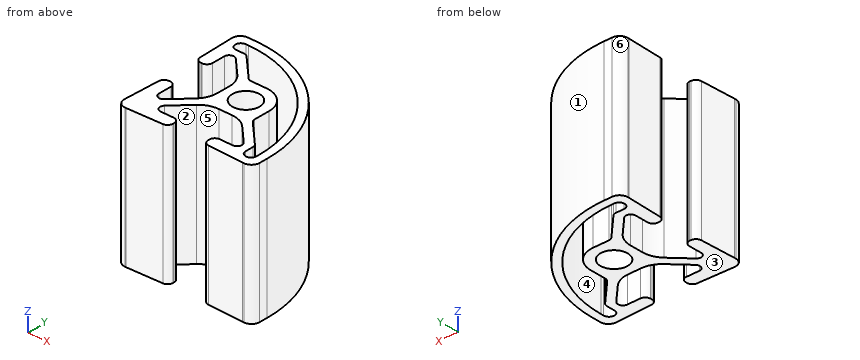
from build123d import *

# Parameters (mm, degrees)
SKETCH1_R      = 2.5
EXTRUDE1_DEPTH = 25.4


with BuildPart() as part:
    # Sketch1 → Extrude1 (new body)
    with BuildSketch(Plane.XY):
        with BuildLine():
            Line((1.22051236, -4.17896), (-1.22051236, -4.17896))
            ThreePointArc((-1.22051236, -4.17896), (-2.846916947, -4.502471987), (-4.22571618, -5.42375618))
            Line((-4.22571618, -5.42375618), (-7.286523897, -8.484563897))
            ThreePointArc((-7.286523897, -8.484563897), (-7.481619373, -9.465375089), (-6.650127794, -10.02096))
            Line((-6.650127794, -10.02096), (-4.24, -10.02096))
            ThreePointArc((-4.24, -10.02096), (-3.532893219, -10.313853219), (-3.24, -11.02096))
            Line((-3.24, -11.02096), (-3.24, -11.272405454))
            ThreePointArc((-3.24, -11.272405454), (-3.5206602, -11.967063824), (-4.205100503, -12.271796281))
            Line((-4.205100503, -12.271796281), (-10.74, -12.5))
            Line((-10.74, -12.5), (-11, -12.5))
            ThreePointArc((-11, -12.5), (-12.060660172, -12.060660172), (-12.5, -11))
            Line((-12.5, -11), (-12.5, -10.74))
            Line((-12.5, -10.74), (-12.271796281, -4.205100503))
            ThreePointArc((-12.271796281, -4.205100503), (-11.967063824, -3.5206602), (-11.272405454, -3.24))
            Line((-11.272405454, -3.24), (-11.02096, -3.24))
            ThreePointArc((-11.02096, -3.24), (-10.313853219, -3.532893219), (-10.02096, -4.24))
            Line((-10.02096, -4.24), (-10.02096, -6.650127794))
            ThreePointArc((-10.02096, -6.650127794), (-9.465375089, -7.481619373), (-8.484563897, -7.286523897))
            Line((-8.484563897, -7.286523897), (-5.42375618, -4.22571618))
            ThreePointArc((-5.42375618, -4.22571618), (-4.502471987, -2.846916947), (-4.17896, -1.22051236))
            Line((-4.17896, -1.22051236), (-4.17896, 1.22051236))
            ThreePointArc((-4.17896, 1.22051236), (-4.502471987, 2.846916947), (-5.42375618, 4.22571618))
            Line((-5.42375618, 4.22571618), (-8.484563897, 7.286523897))
            ThreePointArc((-8.484563897, 7.286523897), (-9.465375089, 7.481619373), (-10.02096, 6.650127794))
            Line((-10.02096, 6.650127794), (-10.02096, 4.24))
            ThreePointArc((-10.02096, 4.24), (-10.313853219, 3.532893219), (-11.02096, 3.24))
            Line((-11.02096, 3.24), (-11.272405454, 3.24))
            ThreePointArc((-11.272405454, 3.24), (-11.967063824, 3.5206602), (-12.271796281, 4.205100503))
            Line((-12.271796281, 4.205100503), (-12.5, 10.74))
            Line((-12.5, 10.74), (-12.5, 11))
            ThreePointArc((-12.5, 11), (-12.060660172, 12.060660172), (-11, 12.5))
            Line((-11, 12.5), (-9.5, 12.5))
            ThreePointArc((-9.5, 12.5), (6.056349186, 6.056349186), (12.5, -9.5))
            Line((12.5, -9.5), (12.5, -11))
            ThreePointArc((12.5, -11), (12.060660172, -12.060660172), (11, -12.5))
            Line((11, -12.5), (10.74, -12.5))
            Line((10.74, -12.5), (4.205100503, -12.271796281))
            ThreePointArc((4.205100503, -12.271796281), (3.5206602, -11.967063824), (3.24, -11.272405454))
            Line((3.24, -11.272405454), (3.24, -11.02096))
            ThreePointArc((3.24, -11.02096), (3.532893219, -10.313853219), (4.24, -10.02096))
            Line((4.24, -10.02096), (6.650127794, -10.02096))
            ThreePointArc((6.650127794, -10.02096), (7.481619373, -9.465375089), (7.286523897, -8.484563897))
            Line((7.286523897, -8.484563897), (4.22571618, -5.42375618))
            ThreePointArc((4.22571618, -5.42375618), (2.846916947, -4.502471987), (1.22051236, -4.17896))
        make_face()
        Circle(SKETCH1_R, mode=Mode.SUBTRACT)
        with BuildLine():
            Line((4.25, 0), (4.25, -2.912506094))
            ThreePointArc((4.25, -2.912506094), (4.326120467, -3.295189526), (4.542893219, -3.619612875))
            Line((4.542893219, -3.619612875), (8.707106781, -7.783826438))
            ThreePointArc((8.707106781, -7.783826438), (8.923879533, -8.108249786), (9, -8.490933219))
            Line((9, -8.490933219), (9, -10))
            ThreePointArc((9, -10), (10, -11), (11, -10))
            Line((11, -10), (11, -9.5))
            ThreePointArc((11, -9.5), (4.995689014, 4.995689014), (-9.5, 11))
            Line((-9.5, 11), (-10, 11))
            ThreePointArc((-10, 11), (-11, 10), (-10, 9))
            Line((-10, 9), (-8.490933219, 9))
            ThreePointArc((-8.490933219, 9), (-8.108249786, 8.923879533), (-7.783826438, 8.707106781))
            Line((-7.783826438, 8.707106781), (-3.619612875, 4.542893219))
            ThreePointArc((-3.619612875, 4.542893219), (-3.295189526, 4.326120467), (-2.912506094, 4.25))
            Line((-2.912506094, 4.25), (0, 4.25))
            ThreePointArc((0, 4.25), (3.00520382, 3.00520382), (4.25, 0))
        make_face(mode=Mode.SUBTRACT)
    extrude(amount=EXTRUDE1_DEPTH)


solid = part.part
The model under review builds one solid part; all positions refer to its coordinate system, in mm. Face numbers are marked on the shaded views. A direction names the side the tool comes from. Coordinates: 2 decimals unless noted, no trailing zeros. Write each loop counter-clockwise with the first axis right and the second up, starting at its lowest first coordinate (ties: lowest second). Pieces come first, ordered by that corner, then holes. Notation, with made-up numbers: (-4.75, 58.5) - (45.25, 58.5) arc R19 cw to (45.25, 69.5) - close; hole circle Ø1 at (-13, -13.75). An arc over 180 degrees is marked (long way). Answer as CSV lines item,"result".
(1) Clearance check with flat-ended pins moving along their axes: pin 1 Ø1.9 at (y, z) = (-6, 13.5) entering from +X; pin 2 Ø0.7 at (y, z) = (5, 11) entering from +X; pin 3 Ø1.9 at (x, z) = (-5, 13) entering from +Y; pin 4 Ø6 at (x, y) = (0, 0) entering from +Z. State where each tip first meets the part, or that it passes through.
Data:
pin 1,"stops at x = 12.35"
pin 2,"stops at x = 7.35"
pin 3,"stops at y = 12.21"
pin 4,"stops at z = 25.4"
(2) We need section B-B (x = -6.25). Give the boundary of the cut face in (y, z).
Data:
outline,"(-12.34, 0) - (-10.02, 0) - (-10.02, 25.4) - (-12.34, 25.4) - close; (-7.45, 0) - (-5.05, 0) - (-5.05, 25.4) - (-7.45, 25.4) - close; (5.05, 0) - (7.17, 0) - (7.17, 25.4) - (5.05, 25.4) - close; (10.74, 0) - (12.26, 0) - (12.26, 25.4) - (10.74, 25.4) - close"
(3) For line 1 along Y through (x, z) = (0, 17); line 2 along X through (y, z) = (-2.25, 23); line 3 along Y through (x, z) = (2.25, 9.5), list the stretches that pass through material, from the lowest coordinate up. Write a range as [from, to].
Data:
line 1,"y = [-4.18, -2.5], [2.5, 4.25], [8.67, 10.34]"
line 2,"x = [-4.31, -1.09], [1.09, 4.25], [9.68, 11.27]"
line 3,"y = [-4.31, -1.09], [1.09, 3.61], [7.3, 9.1]"
(4) We need section A-A (x = -9). Give the boundary of the cut face in (y, z).
Data:
outline,"(-12.44, 0) - (-7.54, 0) - (-7.54, 25.4) - (-12.44, 25.4) - close; (7.54, 0) - (9, 0) - (9, 25.4) - (7.54, 25.4) - close; (10.99, 0) - (12.49, 0) - (12.49, 25.4) - (10.99, 25.4) - close"
(5) Mouldability with a two-part tool opening along Y and no side actions: class the marked faces 1, 2, 3 and 4 as pulls with the +Y half, pulls with the -Y half, needs draft (parallel to the pull), parting line crosses it, or undercut.
Data:
face 1,"pulls with the +Y half"
face 2,"undercut"
face 3,"needs draft"
face 4,"undercut"
(6) We need section D-D (z = 9.5). Count the separate pieces of the cut face and the enclosed holes in it, plus the area to 3 significant figures.
Data:
separate pieces,"1"
enclosed holes,"2"
area,"216 mm2"
(7) We need section C-C (x = 10). Give the boundary of the cut face in (y, z).
Data:
outline,"(-12.47, 0) - (-11, 0) - (-11, 25.4) - (-12.47, 25.4) - close; (-3.18, 0) - (0.69, 0) - (0.69, 25.4) - (-3.18, 25.4) - close"
(8) Tool access review of the marked faces 5 and 6: name each direction out of +Z, -Z, +X, -X, +Y, -Y from which nothing blocks a thin tool from reaching the whole face with its end or side.
Data:
face 5,"+Z, -Z"
face 6,"+Z, -Z, -X, +Y"
